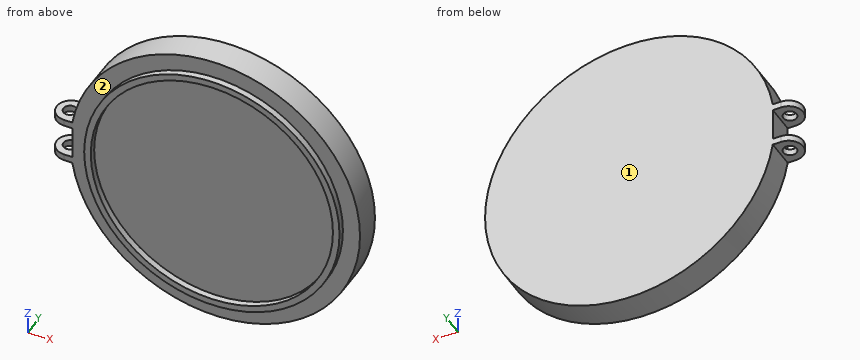
from build123d import *

# Parameters (mm, degrees)
SKETCH3_R           = 1.27
BOSS_EXTRUDE1_DEPTH = 4.445
SKETCH4_W           = 4.419845581
SKETCH4_H           = 6.35
CUT_EXTRUDE1_DEPTH  = 5.588


with BuildPart() as part:
    # Sketch2 → Revolve1 (revolve)
    with BuildSketch(Plane.XY):
        Polygon((0, 0), (0, 5.588), (27.94, 5.588), (27.94, 0), (24.638, 0), (24.638, -1.27), (23.368, -1.27), (23.368, 0), align=None)
    revolve(axis=Axis((0, -1000, 0), (0, 1, 0)))

    # Sketch3 → Boss-Extrude1 (add, symmetric)
    with BuildSketch(Plane.XY):
        with BuildLine():
            Line((-29.21, 0), (-27.305, 0))
            Line((-27.305, 0), (-27.305, 5.588))
            Line((-27.305, 5.588), (-29.21, 5.588))
            ThreePointArc((-29.21, 5.588), (-32.004, 2.794), (-29.21, 0))
        make_face()
        with Locations((-29.464, 2.794)):
            Circle(SKETCH3_R, mode=Mode.SUBTRACT)
    extrude(amount=BOSS_EXTRUDE1_DEPTH, both=True)

    # Sketch4 → Cut-Extrude1 (cut)
    with BuildSketch(Plane(origin=(0, 5.588, 0), x_dir=(1, 0, 0), z_dir=(0, 1, 0))):
        with Locations((-29.79407721, 0)):
            Rectangle(SKETCH4_W, SKETCH4_H)
    extrude(amount=-CUT_EXTRUDE1_DEPTH, mode=Mode.SUBTRACT)


solid = part.part
CAD build for the part. Positions are in the model's coordinates, mm. Face numbers are marked on the shaded views. A direction names the side the tool comes from. Round coordinates to 2 decimals unless told otherwise and drop trailing zeros. Loops run counter-clockwise (first coordinate to the right, second up) from the corner with the lowest first, then second, coordinate; pieces in that order, holes last.
(1) Which spindle directions (+Z, -Z, +X, -X, +Y, -Y) get a long thin tool onto all of the face, cutting with end or side? Do the marked faces 1 and 2. Say none if no direction does.
(2) Drop flat-ended pins along their axis: pin 1 (14 mm diameter, centred on x = 9.5, z = 3, fed in from -Y); pin 2 (1.7 mm diameter, centred on y = 3.5, z = -1, fed in from -X); pin 3 (4 mm diameter, centred on y = 1, z = 8, fed in from -X); pin 4 (1.5 mm diameter, centred on x = -29.464, y = 2.794, fed in from -Z). Give the stop position or say it passes through.
(3) Wall check: line 1 along X through (y, z) = (-0.65, 0); line 2 along Y through (x, z) = (-6, -11.5). Give the ranges that are in metal, low to high.
(4) Cut at B-B (x = 0). Give the cut face in (y, z), plus the area to 3 significant figures.
(5) Cut at A-A (z = 0). Give the cut face in (x, y).
Findings below:
1. face 1: +Z, -Z, +X, -X, +Y
1. face 2: -Y
2. pin 1: stops at y = 0
2. pin 2: stops at x = -27.58
2. pin 3: stops at x = -27.29
2. pin 4: passes through
3. line 1: x = -24.64 to -23.37, 23.37 to 24.64
3. line 2: y = 0 to 5.59
4. outline: (-1.27, -24.64) - (0, -24.64) - (0, -27.94) - (5.59, -27.94) - (5.59, 27.94) - (0, 27.94) - (0, 24.64) - (-1.27, 24.64) - (-1.27, 23.37) - (0, 23.37) - (0, -23.37) - (-1.27, -23.37) - close
4. area: 315 mm2
5. outline: (-27.58, 0) - (-24.64, 0) - (-24.64, -1.27) - (-23.37, -1.27) - (-23.37, 0) - (23.37, 0) - (23.37, -1.27) - (24.64, -1.27) - (24.64, 0) - (27.94, 0) - (27.94, 5.59) - (-27.58, 5.59) - close
